Geometry check sheet. Reference: drawing and pictorial views, mm from the part's lowest x, y, z. A direction names the side the tool comes from. Give positions to 0.01 mm unless a question says otherwise; leave off trailing zeros. Order: outer loops, then holes, each group sorted by start corner. A loop starts at its lowest first (then second) coordinate and runs counter-clockwise, first axis right, second up. Notation, with made-up numbers: (-30, 0.25) - (21, 0.25) arc R19 cw to (21, 7.25) - close; hole circle Ø11 at (-29, 3.25). An arc over 180 degrees is marked (long way). Answer in a Markdown table with one row per item.
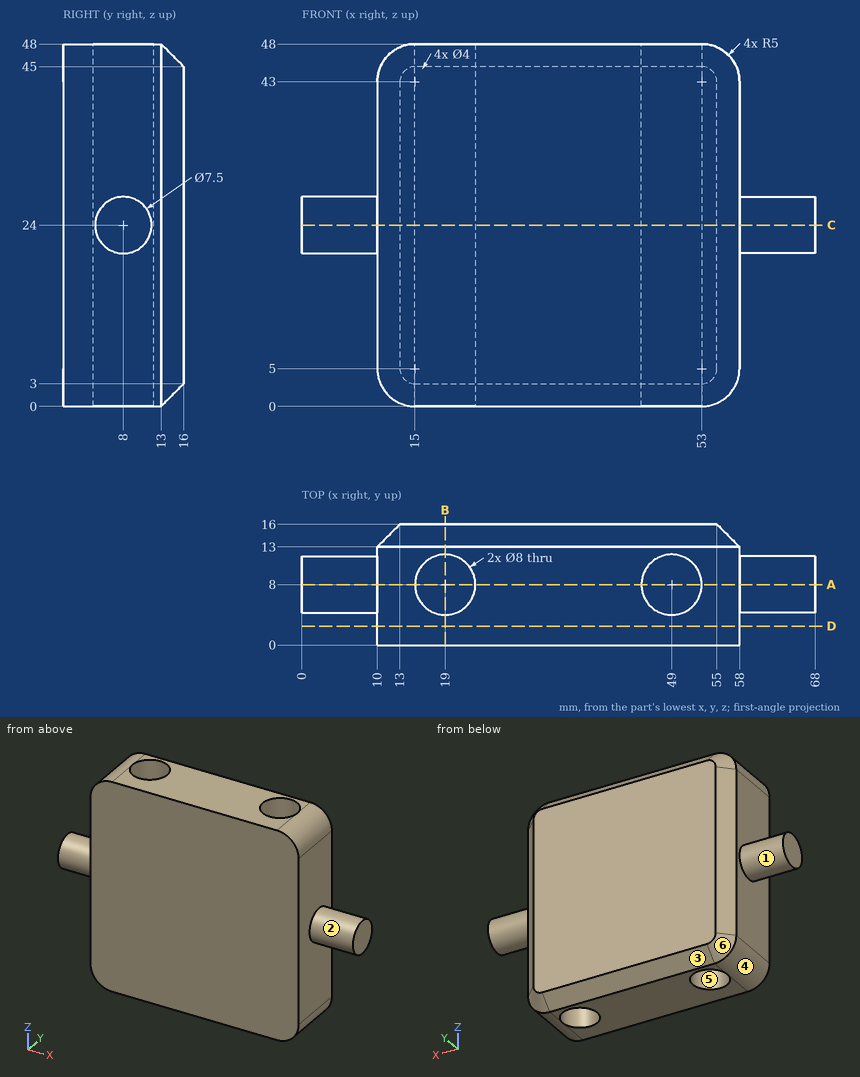
(1) Cross-section at B-B, the plane x = 19. Record the cut outline in (y, z), then the cut area to 3 significant figures.
Geometry says:
| item | result |
|---|---|
| outline | (0, 0) - (4, 0) - (4, 48) - (0, 48) - close; (12, 0) - (13, 0) - (16, 3) - (16, 45) - (13, 48) - (12, 48) - close |
| area | 375 mm² |
(2) Thickness scan on L1, parallel to Y at x = 49, z = 28.5; L2, parallel to X at y = 9, z = 13.5; L3, parallel to X at y = 4.5, z = 22 (1 decimal). Record the ranges inside material, lowest first.
Geometry says:
| item | result |
|---|---|
| L1 | 0 to 4, 12 to 16 |
| L2 | 10 to 15.13, 22.87 to 45.13, 52.87 to 58 |
| L3 | 10 to 17.1, 20.9 to 47.1, 50.9 to 58 |
(3) Mould release check, pull along Y, two halves, no side actions. Record for the marked faces 4, 5 and 6: pulls with the +Y half, pulls with the -Y half, needs draft (parallel to the pull), parting line crosses it, or undercut.
Geometry says:
| item | result |
|---|---|
| face 4 | needs draft |
| face 5 | undercut |
| face 6 | pulls with the +Y half |
(4) Cross-section at A-A, the plane y = 8. Give the number of separate pieces and of enclosed holes in the cut face, then the cut area to 3 significant figures.
Geometry says:
| item | result |
|---|---|
| separate pieces | 3 |
| enclosed holes | 0 |
| area | 1,660 mm² |
(5) Cross-section at C-C, the plane z = 24. Record the cut outline in (x, y).
Geometry says:
| item | result |
|---|---|
| outline | (0, 4.25) - (10, 4.25) - (10, 0) - (58, 0) - (58, 4.25) - (68, 4.25) - (68, 11.75) - (58, 11.75) - (58, 13) - (55, 16) - (13, 16) - (10, 13) - (10, 11.75) - (0, 11.75) - close; hole circle Ø8 at (19, 8); hole circle Ø8 at (49, 8) |
(6) Access from +Z, -Z, +X, -X, +Y, -Y to the whole of each face (thin tool, end or side, straight path). Record for the marked faces 1, 2 and 3.
Geometry says:
| item | result |
|---|---|
| face 1 | -X |
| face 2 | +X |
| face 3 | -Z, +X, -X, +Y |
(7) Cross-section at D-D, the plane y = 2.5. Record the cut outline in (x, z), then the cut area to 3 significant figures.
Geometry says:
| item | result |
|---|---|
| outline | (10, 5) arc R5 ccw to (15, 0) - (53, 0) arc R5 ccw to (58, 5) - (58, 43) arc R5 ccw to (53, 48) - (15, 48) arc R5 ccw to (10, 43) - close |
| area | 2,280 mm² |
(8) Gauge pin test, flat ends, axial feed: P1, Ø3, axis at y = 3.5, z = 21, coming from the +X side; P2, Ø1.5, axis at y = 10.5, z = 6, coming from the -X side. Record the tip position at first contact, or that the pin passes through.
Geometry says:
| item | result |
|---|---|
| P1 | x = 58 |
| P2 | x = 10 |
